Geometry: see drawing. Coordinates: mm, zero at the bounding-box minimum. A direction names the side the tool comes from. Give positions to 0.01 mm unless a question says otherwise; leave off trailing zeros. Loops run counter-clockwise (first coordinate to the right, second up) from the corner with the lowest first, then second, coordinate; pieces in that order, holes last. Notation, with made-up numbers: (22, 39.5) -> (73, 39.5) arc R30 ccw to (73, 78.5) -> close; hole circle Ø5 at (19.5, 51). An arc over 180 degrees is marked (long way). Return JSON: item names as keys, results as strings. Group by question number.
(1) Cut plane D-D on y = 3. Return loops of the section in (x, z).
(2) Ray query, line 1 (Y direction, x = 17, z = 20); line 2 (Z direction, x = 3, y = 1.45); line 3 (X direction, y = 1.65, z = 3). Return the intervals inside material, ascending. Write a range as from..to.
(3) Access query for the marked faces 1 and 2. Directions: +Z, -Z, +X, -X, +Y, -Y. A direction counts if a zero-diameter tool reaches every point of the face in a straight line with its end or side. Return the directions, or none.
(4) Cut plane C-C on y = 5. Return loops of the section in (x, z), then the cut area to 3 significant figures.
(5) Pin query (flat end, axial travel): pin 1 (2 mm diameter, centred on y = 4.5, z = 12, fed in from +X); pin 2 (2 mm diameter, centred on x = 22, z = 12, fed in from +Y); pin 3 (2 mm diameter, centred on x = 22, z = 12.5, fed in from +Y); pin 4 (12 mm diameter, centred on x = 7.5, z = 5, fed in from +Y). Return the tip coordinate at first contact, or that it passes through.
(6) Cut plane A-A on x = 12.5. Give the number of separate pieces and of enclosed holes in the cut face, then the cut area to 3 significant figures.
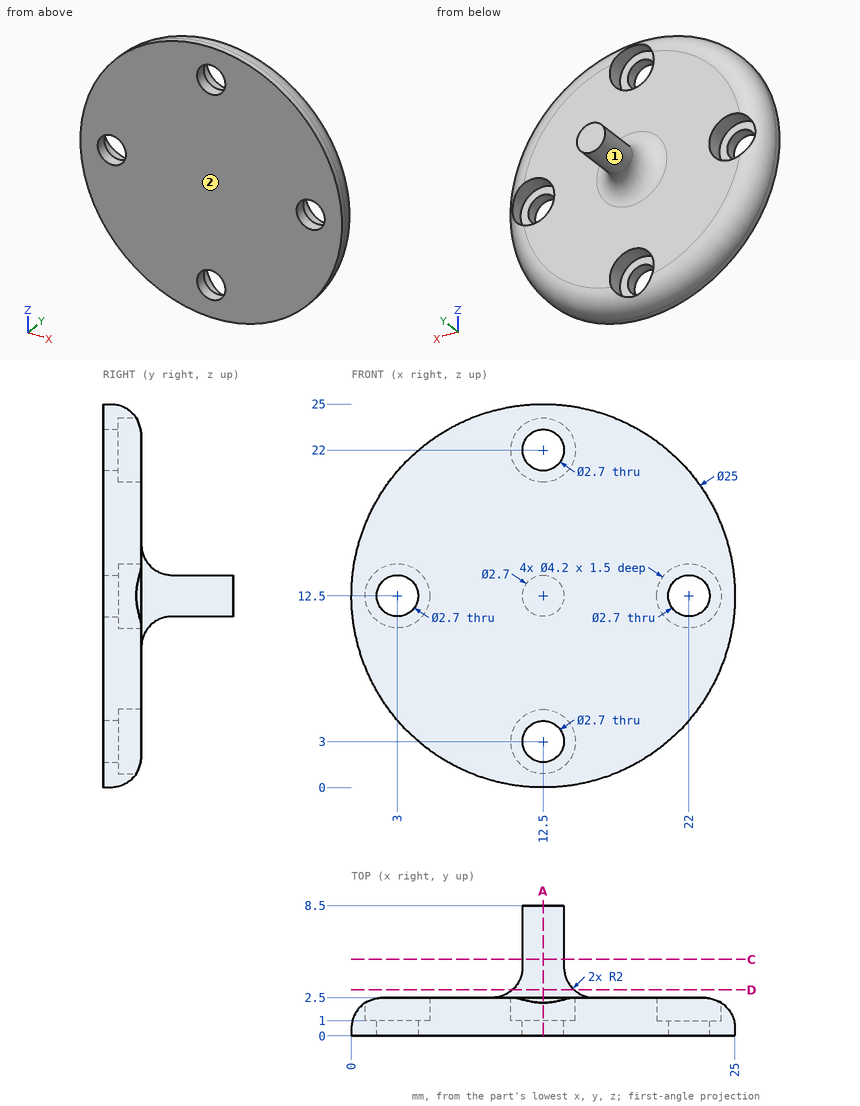
Answers:
{
 "1": {"outline": "circle Ø4.05 at (12.5, 12.5)"},
 "2": {"line 1": "0..2.5", "line 2": "4.75..10.4, 14.6..20.25", "line 3": "4.95..10.4, 14.6..20.05"},
 "3": {"face 1": "+Y", "face 2": "+Z, -Z, +X, -X, -Y"},
 "4": {"outline": "circle Ø2.7 at (12.5, 12.5)", "area": "5.73 mm²"},
 "5": {"pin 1": "x = 14.08", "pin 2": "y = 1", "pin 3": "through", "pin 4": "y = 2.53"},
 "6": {"separate pieces": "3", "enclosed holes": "0", "area": "60.9 mm²"}
}
